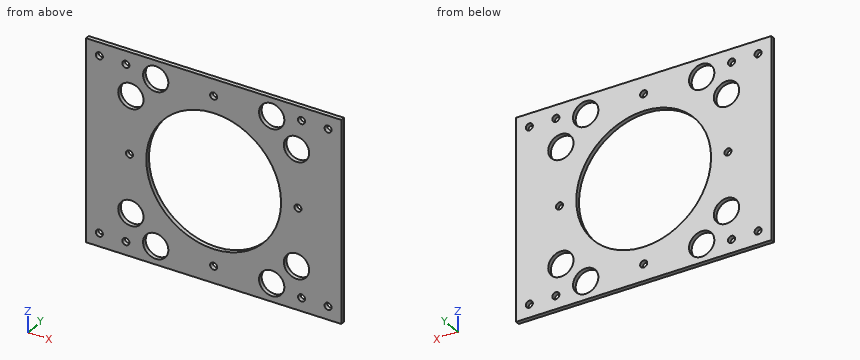
from build123d import *

# Parameters (mm, degrees)
SKETCH2_W           = 152.4
SKETCH2_H           = 152.4
SKETCH2_R           = 50.8
BOSS_EXTRUDE1_DEPTH = 3.175
CUT_EXTRUDE1_REACH  = 109.81
SKETCH3_R           = 2.665000004
CUT_EXTRUDE2_REACH  = 109.81
SKETCH4_R           = 9.525
CUT_EXTRUDE3_REACH  = 109.81
SKETCH5_R           = 2.665000004
SKETCH6_W           = 152.4
SKETCH6_H           = 3.175
BOSS_EXTRUDE2_DEPTH = 20
CUT_EXTRUDE4_REACH  = 124.764
SKETCH7_R           = 2.665000004


with BuildPart() as part:
    # Sketch2 → Boss-Extrude1 (new body)
    with BuildSketch(Plane(origin=(0, 0, 0), x_dir=(1, 0, 0), z_dir=(0, 1, 0))):
        Rectangle(SKETCH2_W, SKETCH2_H)
        with Locations(Location((0, 0, 0), (0, 0, 270))):
            Circle(SKETCH2_R, mode=Mode.SUBTRACT)
    extrude(amount=BOSS_EXTRUDE1_DEPTH)

    # Sketch3 → Cut-Extrude1 (cut, up to next)
    with BuildSketch(Plane(origin=(0, 3.175, 0), x_dir=(1, 0, 0), z_dir=(0, 1, 0)), mode=Mode.PRIVATE) as cut_extrude1_sk1:
        with Locations(Location((-66.2, -66.2, 0), (0, 0, 270))):
            Circle(SKETCH3_R)
    cut_extrude1_tool1 = extrude(cut_extrude1_sk1.sketch, amount=-CUT_EXTRUDE1_REACH, mode=Mode.PRIVATE) & part.part
    # Sketch3 → Cut-Extrude1 (cut, up to next)
    with BuildSketch(Plane(origin=(0, 3.175, 0), x_dir=(1, 0, 0), z_dir=(0, 1, 0)), mode=Mode.PRIVATE) as cut_extrude1_sk2:
        with Locations(Location((-66.2, 66.2, 0), (0, 0, 90))):
            Circle(SKETCH3_R)
    cut_extrude1_tool2 = extrude(cut_extrude1_sk2.sketch, amount=-CUT_EXTRUDE1_REACH, mode=Mode.PRIVATE) & part.part
    # Sketch3 → Cut-Extrude1 (cut, up to next)
    with BuildSketch(Plane(origin=(0, 3.175, 0), x_dir=(1, 0, 0), z_dir=(0, 1, 0)), mode=Mode.PRIVATE) as cut_extrude1_sk3:
        with Locations(Location((66.2, 66.2, 0), (0, 0, 270))):
            Circle(SKETCH3_R)
    cut_extrude1_tool3 = extrude(cut_extrude1_sk3.sketch, amount=-CUT_EXTRUDE1_REACH, mode=Mode.PRIVATE) & part.part
    # Sketch3 → Cut-Extrude1 (cut, up to next)
    with BuildSketch(Plane(origin=(0, 3.175, 0), x_dir=(1, 0, 0), z_dir=(0, 1, 0)), mode=Mode.PRIVATE) as cut_extrude1_sk4:
        with Locations(Location((66.2, -66.2, 0), (0, 0, 90))):
            Circle(SKETCH3_R)
    cut_extrude1_tool4 = extrude(cut_extrude1_sk4.sketch, amount=-CUT_EXTRUDE1_REACH, mode=Mode.PRIVATE) & part.part
    add(cut_extrude1_tool1.solids().sort_by_distance((-66.2, 3.175, 66.2))[0], mode=Mode.SUBTRACT)
    add(cut_extrude1_tool2.solids().sort_by_distance((-66.2, 3.175, -66.2))[0], mode=Mode.SUBTRACT)
    add(cut_extrude1_tool3.solids().sort_by_distance((66.2, 3.175, -66.2))[0], mode=Mode.SUBTRACT)
    add(cut_extrude1_tool4.solids().sort_by_distance((66.2, 3.175, 66.2))[0], mode=Mode.SUBTRACT)

    # Sketch4 → Cut-Extrude2 (cut, up to next)
    with BuildSketch(Plane(origin=(0, 3.175, 0), x_dir=(1, 0, 0), z_dir=(0, 1, 0)), mode=Mode.PRIVATE) as cut_extrude2_sk1:
        with Locations(Location((62.419385775, -43.70652445, 0), (0, 0, 270))):
            Circle(SKETCH4_R)
    cut_extrude2_tool1 = extrude(cut_extrude2_sk1.sketch, amount=-CUT_EXTRUDE2_REACH, mode=Mode.PRIVATE) & part.part
    # Sketch4 → Cut-Extrude2 (cut, up to next)
    with BuildSketch(Plane(origin=(0, 3.175, 0), x_dir=(1, 0, 0), z_dir=(0, 1, 0)), mode=Mode.PRIVATE) as cut_extrude2_sk2:
        with Locations(Location((43.70652445, -62.419385775, 0), (0, 0, 270))):
            Circle(SKETCH4_R)
    cut_extrude2_tool2 = extrude(cut_extrude2_sk2.sketch, amount=-CUT_EXTRUDE2_REACH, mode=Mode.PRIVATE) & part.part
    # Sketch4 → Cut-Extrude2 (cut, up to next)
    with BuildSketch(Plane(origin=(0, 3.175, 0), x_dir=(1, 0, 0), z_dir=(0, 1, 0)), mode=Mode.PRIVATE) as cut_extrude2_sk3:
        with Locations(Location((43.70652445, 62.419385775, 0), (0, 0, 90))):
            Circle(SKETCH4_R)
    cut_extrude2_tool3 = extrude(cut_extrude2_sk3.sketch, amount=-CUT_EXTRUDE2_REACH, mode=Mode.PRIVATE) & part.part
    # Sketch4 → Cut-Extrude2 (cut, up to next)
    with BuildSketch(Plane(origin=(0, 3.175, 0), x_dir=(1, 0, 0), z_dir=(0, 1, 0)), mode=Mode.PRIVATE) as cut_extrude2_sk4:
        with Locations(Location((62.419385775, 43.70652445, 0), (0, 0, 90))):
            Circle(SKETCH4_R)
    cut_extrude2_tool4 = extrude(cut_extrude2_sk4.sketch, amount=-CUT_EXTRUDE2_REACH, mode=Mode.PRIVATE) & part.part
    # Sketch4 → Cut-Extrude2 (cut, up to next)
    with BuildSketch(Plane(origin=(0, 3.175, 0), x_dir=(1, 0, 0), z_dir=(0, 1, 0)), mode=Mode.PRIVATE) as cut_extrude2_sk5:
        with Locations(Location((-43.70652445, 62.419385775, 0), (0, 0, 270))):
            Circle(SKETCH4_R)
    cut_extrude2_tool5 = extrude(cut_extrude2_sk5.sketch, amount=-CUT_EXTRUDE2_REACH, mode=Mode.PRIVATE) & part.part
    # Sketch4 → Cut-Extrude2 (cut, up to next)
    with BuildSketch(Plane(origin=(0, 3.175, 0), x_dir=(1, 0, 0), z_dir=(0, 1, 0)), mode=Mode.PRIVATE) as cut_extrude2_sk6:
        with Locations(Location((-62.419385775, 43.70652445, 0), (0, 0, 270))):
            Circle(SKETCH4_R)
    cut_extrude2_tool6 = extrude(cut_extrude2_sk6.sketch, amount=-CUT_EXTRUDE2_REACH, mode=Mode.PRIVATE) & part.part
    # Sketch4 → Cut-Extrude2 (cut, up to next)
    with BuildSketch(Plane(origin=(0, 3.175, 0), x_dir=(1, 0, 0), z_dir=(0, 1, 0)), mode=Mode.PRIVATE) as cut_extrude2_sk7:
        with Locations(Location((-43.70652445, -62.419385775, 0), (0, 0, 90))):
            Circle(SKETCH4_R)
    cut_extrude2_tool7 = extrude(cut_extrude2_sk7.sketch, amount=-CUT_EXTRUDE2_REACH, mode=Mode.PRIVATE) & part.part
    # Sketch4 → Cut-Extrude2 (cut, up to next)
    with BuildSketch(Plane(origin=(0, 3.175, 0), x_dir=(1, 0, 0), z_dir=(0, 1, 0)), mode=Mode.PRIVATE) as cut_extrude2_sk8:
        with Locations(Location((-62.419385775, -43.70652445, 0), (0, 0, 90))):
            Circle(SKETCH4_R)
    cut_extrude2_tool8 = extrude(cut_extrude2_sk8.sketch, amount=-CUT_EXTRUDE2_REACH, mode=Mode.PRIVATE) & part.part
    add(cut_extrude2_tool1.solids().sort_by_distance((62.419386, 3.175, 43.706524))[0], mode=Mode.SUBTRACT)
    add(cut_extrude2_tool2.solids().sort_by_distance((43.706524, 3.175, 62.419386))[0], mode=Mode.SUBTRACT)
    add(cut_extrude2_tool3.solids().sort_by_distance((43.706524, 3.175, -62.419386))[0], mode=Mode.SUBTRACT)
    add(cut_extrude2_tool4.solids().sort_by_distance((62.419386, 3.175, -43.706524))[0], mode=Mode.SUBTRACT)
    add(cut_extrude2_tool5.solids().sort_by_distance((-43.706524, 3.175, -62.419386))[0], mode=Mode.SUBTRACT)
    add(cut_extrude2_tool6.solids().sort_by_distance((-62.419386, 3.175, -43.706524))[0], mode=Mode.SUBTRACT)
    add(cut_extrude2_tool7.solids().sort_by_distance((-43.706524, 3.175, 62.419386))[0], mode=Mode.SUBTRACT)
    add(cut_extrude2_tool8.solids().sort_by_distance((-62.419386, 3.175, 43.706524))[0], mode=Mode.SUBTRACT)

    # Sketch5 → Cut-Extrude3 (cut, up to next)
    with BuildSketch(Plane(origin=(0, 3.175, 0), x_dir=(1, 0, 0), z_dir=(0, 1, 0)), mode=Mode.PRIVATE) as cut_extrude3_sk1:
        with Locations(Location((0, -63.5, 0), (0, 0, 270))):
            Circle(SKETCH5_R)
    cut_extrude3_tool1 = extrude(cut_extrude3_sk1.sketch, amount=-CUT_EXTRUDE3_REACH, mode=Mode.PRIVATE) & part.part
    # Sketch5 → Cut-Extrude3 (cut, up to next)
    with BuildSketch(Plane(origin=(0, 3.175, 0), x_dir=(1, 0, 0), z_dir=(0, 1, 0)), mode=Mode.PRIVATE) as cut_extrude3_sk2:
        with Locations(Location((-63.5, 0, 0), (0, 0, 270))):
            Circle(SKETCH5_R)
    cut_extrude3_tool2 = extrude(cut_extrude3_sk2.sketch, amount=-CUT_EXTRUDE3_REACH, mode=Mode.PRIVATE) & part.part
    # Sketch5 → Cut-Extrude3 (cut, up to next)
    with BuildSketch(Plane(origin=(0, 3.175, 0), x_dir=(1, 0, 0), z_dir=(0, 1, 0)), mode=Mode.PRIVATE) as cut_extrude3_sk3:
        with Locations(Location((0, 63.5, 0), (0, 0, 270))):
            Circle(SKETCH5_R)
    cut_extrude3_tool3 = extrude(cut_extrude3_sk3.sketch, amount=-CUT_EXTRUDE3_REACH, mode=Mode.PRIVATE) & part.part
    # Sketch5 → Cut-Extrude3 (cut, up to next)
    with BuildSketch(Plane(origin=(0, 3.175, 0), x_dir=(1, 0, 0), z_dir=(0, 1, 0)), mode=Mode.PRIVATE) as cut_extrude3_sk4:
        with Locations(Location((63.5, 0, 0), (0, 0, 270))):
            Circle(SKETCH5_R)
    cut_extrude3_tool4 = extrude(cut_extrude3_sk4.sketch, amount=-CUT_EXTRUDE3_REACH, mode=Mode.PRIVATE) & part.part
    add(cut_extrude3_tool1.solids().sort_by_distance((0, 3.175, 63.5))[0], mode=Mode.SUBTRACT)
    add(cut_extrude3_tool2.solids().sort_by_distance((-63.5, 3.175, 0))[0], mode=Mode.SUBTRACT)
    add(cut_extrude3_tool3.solids().sort_by_distance((0, 3.175, -63.5))[0], mode=Mode.SUBTRACT)
    add(cut_extrude3_tool4.solids().sort_by_distance((63.5, 3.175, 0))[0], mode=Mode.SUBTRACT)

    # Sketch6 → Boss-Extrude2 (add)
    with BuildSketch(Plane(origin=(76.2, 0, 0), x_dir=(0, 0, -1), z_dir=(1, 0, 0))):
        with Locations((0, 1.5875)):
            Rectangle(SKETCH6_W, SKETCH6_H)
    boss_extrude2 = extrude(amount=BOSS_EXTRUDE2_DEPTH)

    # Sketch7 → Cut-Extrude4 (cut, up to next)
    with BuildSketch(Plane(origin=(0, 3.175, 0), x_dir=(1, 0, 0), z_dir=(0, 1, 0)), mode=Mode.PRIVATE) as cut_extrude4_sk1:
        with Locations(Location((86.2, -66.2, 0), (0, 0, 270))):
            Circle(SKETCH7_R)
    cut_extrude4_tool1 = extrude(cut_extrude4_sk1.sketch, amount=-CUT_EXTRUDE4_REACH, mode=Mode.PRIVATE) & part.part
    # Sketch7 → Cut-Extrude4 (cut, up to next)
    with BuildSketch(Plane(origin=(0, 3.175, 0), x_dir=(1, 0, 0), z_dir=(0, 1, 0)), mode=Mode.PRIVATE) as cut_extrude4_sk2:
        with Locations(Location((86.2, 66.2, 0), (0, 0, 270))):
            Circle(SKETCH7_R)
    cut_extrude4_tool2 = extrude(cut_extrude4_sk2.sketch, amount=-CUT_EXTRUDE4_REACH, mode=Mode.PRIVATE) & part.part
    cut_extrude4_1 = cut_extrude4_tool1.solids().sort_by_distance((86.2, 3.175, 66.2))[0]
    add(cut_extrude4_1, mode=Mode.SUBTRACT)
    cut_extrude4_2 = cut_extrude4_tool2.solids().sort_by_distance((86.2, 3.175, -66.2))[0]
    add(cut_extrude4_2, mode=Mode.SUBTRACT)
    cut_extrude4 = cut_extrude4_1 + cut_extrude4_2  # Cut-Extrude4 as one shape, for the pattern or mirror that repeats it

    # Mirror1: Boss-Extrude2, Cut-Extrude4 across plane
    add(boss_extrude2.mirror(Plane(origin=(0, 0, 0), x_dir=(0, 0, 1), z_dir=(1, 0, 0))))
    add(cut_extrude4.mirror(Plane(origin=(0, 0, 0), x_dir=(0, 0, 1), z_dir=(1, 0, 0))), mode=Mode.SUBTRACT)


solid = part.part
For this review, take the finished solid that the model builds, in its own axes (mm). Give positions to 0.01 mm unless a question says otherwise; leave off trailing zeros. Order: outer loops, then holes, each group sorted by start corner. A loop starts at its lowest first (then second) coordinate and runs counter-clockwise, first axis right, second up. Notation, with made-up numbers: (43, 41) - (50, 41) arc R13 cw to (50, 51) - close; hole circle Ø1 at (15.25, 34.5). An arc over 180 degrees is marked (long way). Answer as a JSON object with one key per item and string values. Group by question number.
Item 1: Wall thickness on line 1 along Z through (x, y) = (63, 1.2); line 2 along X through (y, z) = (1.3, -52); line 3 along Z through (x, y) = (-68, 2.55): over which ranges is each line inside the solid? List them lowest first.
Item 2: Take a section at C-C on z = 16. Give the boundary of the cut face in (x, y) (3 decimals).
Item 3: Take a section at D-D on y = 1. Give the number of separate pieces and of enclosed holes in the cut face, and give its area (3 significant figures).
Item 4: Take a section at A-A on z = 0. Give the boundary of the cut face in (x, y) (3 decimals).
Item 5: Take a section at B-B on x = 0. Give the boundary of the cut face in (y, z) (3 decimals), and give its area (3 significant figures).
Reported:
{
 "1": {"line 1": "-76.2 to -53.21, -34.2 to -2.62, 2.62 to 34.2, 53.21 to 76.2", "line 2": "-96.2 to -67.1, -57.73 to 57.73, 67.1 to 96.2", "line 3": "-76.2 to -68.17, -64.23 to -51.43, -35.99 to 35.99, 51.43 to 64.23, 68.17 to 76.2"},
 "2": {"outline": "(-96.2, 0) - (-48.215, 0) - (-48.215, 3.175) - (-96.2, 3.175) - close; (48.215, 0) - (96.2, 0) - (96.2, 3.175) - (48.215, 3.175) - close"},
 "3": {"separate pieces": "1", "enclosed holes": "21", "area": "18,700 mm^2"},
 "4": {"outline": "(-96.2, 0) - (-66.165, 0) - (-66.165, 3.175) - (-96.2, 3.175) - close; (-60.835, 0) - (-50.8, 0) - (-50.8, 3.175) - (-60.835, 3.175) - close; (50.8, 0) - (60.835, 0) - (60.835, 3.175) - (50.8, 3.175) - close; (66.165, 0) - (96.2, 0) - (96.2, 3.175) - (66.165, 3.175) - close"},
 "5": {"outline": "(0, -76.2) - (3.175, -76.2) - (3.175, -66.165) - (0, -66.165) - close; (0, -60.835) - (3.175, -60.835) - (3.175, -50.8) - (0, -50.8) - close; (0, 50.8) - (3.175, 50.8) - (3.175, 60.835) - (0, 60.835) - close; (0, 66.165) - (3.175, 66.165) - (3.175, 76.2) - (0, 76.2) - close", "area": "127 mm^2"}
}
